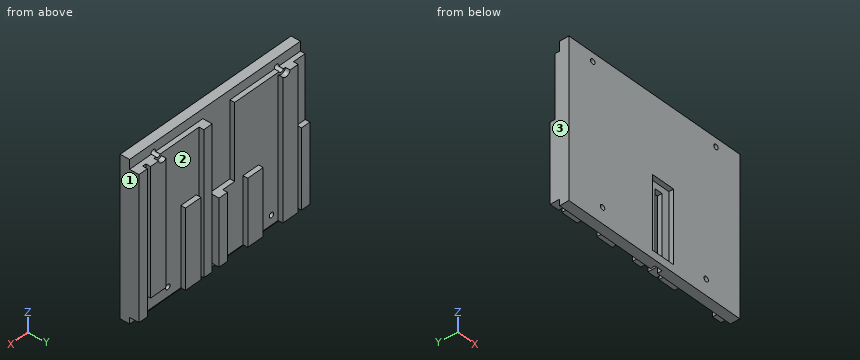
from build123d import *

# Parameters (mm, degrees)
SKETCH1_W           = 122
SKETCH1_H           = 100
BOSS_EXTRUDE1_DEPTH = 3
SKETCH2_W           = 5
SKETCH2_H           = 47
CUT_EXTRUDE1_DEPTH  = 4
SKETCH3_W           = 52.3
SKETCH3_H           = 90
BOSS_EXTRUDE2_DEPTH = 3
SKETCH4_W           = 6
SKETCH4_H           = 50
SKETCH4_W_2         = 11
SKETCH4_H_2         = 90
SKETCH4_H_3         = 42
SKETCH4_H_4         = 80
BOSS_EXTRUDE3_DEPTH = 3
SKETCH7_W           = 122
SKETCH7_H           = 100
SKETCH7_W_2         = 14.9
SKETCH7_H_2         = 46
BOSS_EXTRUDE5_DEPTH = 3
SKETCH8_R           = 1.6
CUT_EXTRUDE2_DEPTH  = 13
CUT_EXTRUDE3_START  = 3
SKETCH9_R           = 3
CUT_EXTRUDE3_DEPTH  = 4


with BuildPart() as part:
    # Sketch1 → Boss-Extrude1 (new body)
    with BuildSketch(Plane(origin=(0, 0, 0), x_dir=(1, 0, 0), z_dir=(0, 1, 0))):
        with Locations((61, 50)):
            Rectangle(SKETCH1_W, SKETCH1_H)
    extrude(amount=BOSS_EXTRUDE1_DEPTH)

    # Sketch2 → Cut-Extrude1 (cut, through all)
    with BuildSketch(Plane(origin=(0, 3, 0), x_dir=(1, 0, 0), z_dir=(0, 1, 0))):
        with Locations((67.3, 76.5)):
            Rectangle(SKETCH2_W, SKETCH2_H)
    extrude(amount=-CUT_EXTRUDE1_DEPTH, mode=Mode.SUBTRACT)

    # Sketch3 → Boss-Extrude2 (add)
    with BuildSketch(Plane(origin=(0, 3, 0), x_dir=(1, 0, 0), z_dir=(0, 1, 0))):
        Polygon((0, 96), (64.8, 96), (64.8, 54), (50.3, 54), (50.3, 6), (0, 6), align=None)
        with Locations((95.85, 51)):
            Rectangle(SKETCH3_W, SKETCH3_H)
    extrude(amount=BOSS_EXTRUDE2_DEPTH)

    # Sketch4 → Boss-Extrude3 (add)
    with BuildSketch(Plane(origin=(0, 6, 0), x_dir=(1, 0, 0), z_dir=(0, 1, 0))):
        with Locations((3, 71)):
            Rectangle(SKETCH4_W, SKETCH4_H)
        with Locations((13.8, 51)):
            Rectangle(SKETCH4_W_2, SKETCH4_H_2)
        with Locations((38.8, 75)):
            Rectangle(SKETCH4_W_2, SKETCH4_H_3)
        with Locations((61.8, 75)):
            Rectangle(SKETCH4_W, SKETCH4_H_3)
        with Locations((83.2, 71)):
            Rectangle(SKETCH4_W_2, SKETCH4_H)
        with Locations((108.2, 46)):
            Rectangle(SKETCH4_W_2, SKETCH4_H_4)
        with Locations((119, 51)):
            Rectangle(SKETCH4_W, SKETCH4_H_2)
        with Locations((72.7, 51)):
            Rectangle(SKETCH4_W, SKETCH4_H_2)
    extrude(amount=BOSS_EXTRUDE3_DEPTH)

    # Sketch7 → Boss-Extrude5 (add)
    with BuildSketch(Plane.XZ):
        with Locations((61, -50)):
            Rectangle(SKETCH7_W, SKETCH7_H)
        with Locations((67.25, -72)):
            Rectangle(SKETCH7_W_2, SKETCH7_H_2, mode=Mode.SUBTRACT)
    extrude(amount=BOSS_EXTRUDE5_DEPTH)

    # Sketch8 → Cut-Extrude2 (cut, through all)
    with BuildSketch(Plane.XZ.offset(3)):
        with Locations((105, -5.5)):
            Circle(SKETCH8_R)
        with Locations((17, -5.5)):
            Circle(SKETCH8_R)
        with Locations((24, -90)):
            Circle(SKETCH8_R)
        with Locations((98, -90)):
            Circle(SKETCH8_R)
    extrude(amount=-CUT_EXTRUDE2_DEPTH, mode=Mode.SUBTRACT)

    # Sketch9 → Cut-Extrude3 (cut, through all)
    with BuildSketch(Plane(origin=(0, 3, 0), x_dir=(1, 0, 0), z_dir=(0, 1, 0)).offset(CUT_EXTRUDE3_START)):
        with Locations((17, 5.5)):
            Circle(SKETCH9_R)
        with Locations((105, 5.5)):
            Circle(SKETCH9_R)
    extrude(amount=CUT_EXTRUDE3_DEPTH, mode=Mode.SUBTRACT)


solid = part.part
Work out the finished part from the listing and answer in its coordinate system (mm). Face numbers are marked on the shaded views. Round coordinates to 2 decimals unless told otherwise and drop trailing zeros. Write each loop counter-clockwise with the first axis right and the second up, starting at its lowest first coordinate (ties: lowest second). Pieces come first, ordered by that corner, then holes. Notation, with made-up numbers: (34.25, 86) - (86.25, 86) arc R26 ccw to (86.25, 100) - close; hole circle Ø7 at (-21, 44). An arc over 180 degrees is marked (long way). Answer in a Markdown table with one row per item. Add a question column.
1. Given pin 1 (1.5 mm diameter, centred on x = 108, y = 7, fed in from -Z); pin 2 (1.5 mm diameter, centred on x = 66, y = 2.5, fed in from -Z); pin 3 (1.9 mm diameter, centred on x = 24, z = -90, fed in from +Y); pin 4 (1.5 mm diameter, centred on x = 85.5, y = 8, fed in from +Z), each flat-ended and moving along its own axis, determine where each tip first touches the part or whether it passes through.
2. Find the intervals of material crossed by line 1 along X through (y, z) = (8, -52); line 2 along X through (y, z) = (2, -90); line 3 along X through (y, z) = (7.5, -39.5), in increasing order. Write a range as from..to.
3. A cutting plane is placed at C-C, the plane x = 30.5. Determine the outline of the cut face in (y, z).
4. The mould has two halves that part along X. Classify the marked faces 1, 2 and 3: +X half, -X half, draft (parallel to the pull), parting line (faces both ways), or undercut.
5. A cutting plane is placed at D-D, the plane z = -37. Determine the outline of the cut face in (x, y).
6. A cutting plane is placed at B-B, the plane y = 7.5. Count the separate pieces of the cut face and the enclosed holes in it, and give its area (3 significant figures).
7. A cutting plane is placed at A-A, the plane x = 105. Determine the outline of the cut face in (y, z).
Worked out:
| question | item | result |
|---|---|---|
| 1 | pin 1 | z = -86 |
| 1 | pin 2 | z = -53 |
| 1 | pin 3 | through |
| 1 | pin 4 | z = -46 |
| 2 | line 1 | 0..6, 8.3..19.3, 69.7..75.7, 77.7..88.7, 102.7..113.7, 116..122 |
| 2 | line 2 | 0..22.4, 25.6..64.8, 69.8..96.4, 99.6..122 |
| 2 | line 3 | 8.3..19.3, 69.7..75.7, 102.7..113.7, 116..122 |
| 3 | outline | (-3, -100) - (3, -100) - (3, -96) - (6, -96) - (6, -6) - (3, -6) - (3, 0) - (-3, 0) - close |
| 4 | face 1 | +X half |
| 4 | face 2 | undercut |
| 4 | face 3 | -X half |
| 5 | outline | (0, -3) - (122, -3) - (122, 9) - (116, 9) - (116, 6) - (113.7, 6) - (113.7, 9) - (102.7, 9) - (102.7, 6) - (75.7, 6) - (75.7, 9) - (69.7, 9) - (69.7, 3) - (50.3, 3) - (50.3, 6) - (19.3, 6) - (19.3, 9) - (8.3, 9) - (8.3, 6) - (0, 6) - close |
| 6 | separate pieces | 8 |
| 6 | enclosed holes | 0 |
| 6 | area | 4,490 mm^2 |
| 7 | outline | (-3, -100) - (3, -100) - (3, -96) - (6, -96) - (6, -86) - (9, -86) - (9, -8.5) - (6, -8.5) - (6, -7.1) - (-3, -7.1) - close; (-3, -3.9) - (3, -3.9) - (3, 0) - (-3, 0) - close |
